Autodesk Inventor part; units mm, degrees
ref_plane "YZ Plane" through (0, 0, 0) normal (1, 0, 0) x (0, 1, 0)
ref_plane "XZ Plane" through (0, 0, 0) normal (0, 1, 0) x (-1, 0, 0)
ref_plane "XY Plane" through (0, 0, 0) normal (0, 0, 1) x (1, 0, 0)
sketch "스케치1" plane through (0, 0, 0) normal (0, 0, 1) x (1, 0, 0)
  circle A0 centre (0.4717, -6.8619) radius 1.3
  circle A1 centre (0.4717, 3.0376) radius 1.3
  circle A2 centre (-9.4278, 3.0376) radius 1.3
  circle A3 centre (-9.4278, -6.8619) radius 1.3
  circle A4 centre (-4.4781, -1.9122) radius 10
  circle A5 centre (-4.4781, -1.9122) radius 5.5
  circle A6 centre (-4.4781, -1.9122) radius 10
  circle A7 centre (0.4717, -6.8619) radius 1.3
  circle A8 centre (0.4717, 3.0376) radius 1.3
  circle A9 centre (-9.4278, 3.0376) radius 1.3
  circle A10 centre (-9.4278, -6.8619) radius 1.3
  point P0 (0, 0)
  dimension "d6" = 20
  dimension "d7" = 11
  dimension "d8" = 2.6
  dimension "d9" = 2.6
  dimension "d10" = 2.6
  dimension "d11" = 2.6
extrude "돌출1" add sketch "스케치1" along normal blind 2.3 contours A4 | A5
sketch "스케치2" plane through (-4.4781, -1.9122, 2.3) normal (0, 0, 1) x (1, 0, 0)
  circle A0 centre (0, 0) radius 10
  circle A1 centre (0, 0) radius 3
  circle A2 centre (0, 0) radius 2.5
  dimension "d2" = 6
  dimension "d5" = 5
extrude "돌출2" add sketch "스케치2" along normal blind 4.5 contours A1
properties part number "pitch_motor1" material "고무, 검은색"
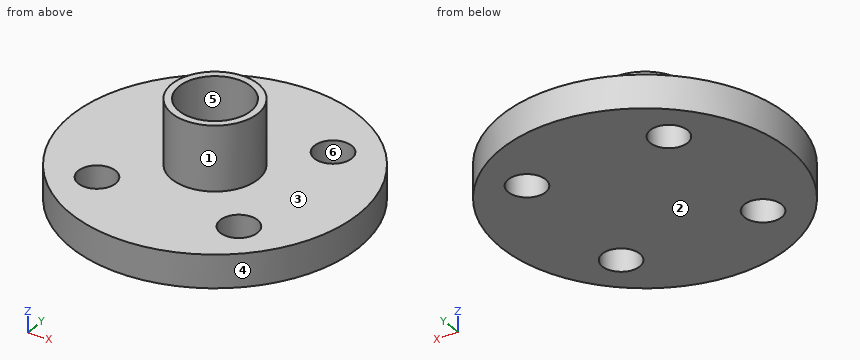
The listing builds one solid part. Answer for the finished solid, in the listing's coordinates (mm). Face numbers are marked on the shaded views. A direction names the side the tool comes from. Round coordinates to 2 decimals unless told otherwise and drop trailing zeros. Order: outer loops, then holes, each group sorted by start corner. A loop starts at its lowest first (then second) coordinate and runs counter-clockwise, first axis right, second up. Notation, with made-up numbers: (-18, 9.25) - (13, 9.25) arc R17 ccw to (13, 15.25) - close; hole circle Ø3 at (13.25, 41). An arc over 180 degrees is marked (long way). Put each result on its own line as item: value. Start each with the question number.
(1) Straight lines are drawn through the part: probe 1 along X at (y, z) = (3.75, 1.5); probe 2 along X at (y, z) = (-7.5, 2); probe 3 along Z at (x, y) = (-2.25, -6.75). For each, find the intervals that lie inside material, in ascending order. Write a range as from..to.
(2) Find section B-B (y = 2.75). Give the vertices of the cut face in (x, z).
(3) Find section D-D (z = 1.75). Give the vertices of the cut face in (x, y), plus the area to 3 significant figures.
(4) Find section A-A (x = -0.25). Give the vertices of the cut face in (y, z), plus the area to 3 significant figures.
(5) Determine the mould class of the marked faces 3, 4, 5 and 6 for opening direction X: released by +X, released by -X, zero draft, split by the parting line, or undercut.
(6) Given P1, Ø1, axis at y = -0.5, z = 2, coming from the -X side; P2, Ø3, axis at x = 0.47, y = 3.04, coming from the -Z side; P3, Ø4, axis at x = -4.48, y = -1.91, coming from the +Z side; P4, Ø2, axis at x = 0.47, y = -6.86, coming from the -Z side, each flat-ended and moving along its own axis, determine where each tip first touches the part or whether it passes through.
(7) Find section C-C (y = -1). Give the vertices of the cut face in (x, z), plus the area to 3 significant figures.
(8) For the marked faces 1 and 2, determine the directions among +Z, -Z, +X, -X, +Y, -Y from which every point of the face is accessible in a straight line to the end or side of a thin tool.
Reply:
1. probe 1: -12.72..-10.52, -8.34..-0.62, 1.56..3.76
1. probe 2: -12.77..-10.56, -8.3..-0.66, 1.6..3.82
1. probe 3: 0..2.3
2. outline: (-13.32, 0) - (-10.7, 0) - (-10.7, 2.3) - (-13.32, 2.3) - close; (-8.16, 0) - (-0.8, 0) - (-0.8, 2.3) - (-8.16, 2.3) - close; (1.74, 0) - (4.37, 0) - (4.37, 2.3) - (1.74, 2.3) - close
3. outline: circle Ø20 at (-4.48, -1.91); hole circle Ø2.6 at (-9.43, -6.86); hole circle Ø2.6 at (-9.43, 3.04); hole circle Ø2.6 at (0.47, -6.86); hole circle Ø2.6 at (0.47, 3.04)
3. area: 293 mm^2
4. outline: (-10.97, 0) - (-7.94, 0) - (-7.94, 2.3) - (-10.97, 2.3) - close; (-5.78, 0) - (1.96, 0) - (1.96, 2.3) - (-5.78, 2.3) - close; (4.12, 0) - (7.15, 0) - (7.15, 2.3) - (4.12, 2.3) - close
4. area: 31.7 mm^2
5. face 3: zero draft
5. face 4: split by the parting line
5. face 5: undercut
5. face 6: undercut
6. P1: x = -14.44
6. P2: z = 0
6. P3: z = 2.3
6. P4: through
7. outline: (-14.44, 0) - (5.48, 0) - (5.48, 2.3) - (-1.62, 2.3) - (-1.62, 6.8) - (-2.15, 6.8) - (-2.15, 2.3) - (-6.81, 2.3) - (-6.81, 6.8) - (-7.34, 6.8) - (-7.34, 2.3) - (-14.44, 2.3) - close
7. area: 50.6 mm^2
8. face 1: +Z
8. face 2: -Z, +X, -X, +Y, -Y
